from build123d import *

# Parameters (mm, degrees)
F1_DEPTH = 20


with BuildPart() as f1:
    # F0 (on Top) → F1 (new body)
    with BuildSketch(Plane.XY):
        Polygon((1.5, 50), (-1.5, 50), (-1.5, 47), (-1.5, -50), (1.5, -50), (1.5, 27), (51.5, 27), (51.5, 30), (51.5, 50), (48.5, 50), (48.5, 30), (28.5, 30), (28.5, 50), (25.5, 50), (25.5, 30), (1.5, 30), align=None)
    extrude(amount=-F1_DEPTH)

    # F3: sweep along a path in F2
    with BuildLine(Plane(origin=(-1.5, 0, 0), x_dir=(0, -1, 0), z_dir=(-1, 0, 0))) as f3_path:
        Line((-48.5, 0), (-43.5, -20))
    # F0 (on Top) → F3 (sweep)
    with BuildSketch(Plane.XY):
        Polygon((-1.5, 47), (-1.5, 50), (-12, 50), (-12, 47), (-12, 41), (-9, 41), (-5, 41), (-5, 43.5), (-9, 43.5), (-9, 47), align=None)
    sweep(path=f3_path.line)


solid = f1.part
CAD build for the part. Positions are in the model's coordinates, mm. A direction names the side the tool comes from. Round coordinates to 2 decimals unless told otherwise and drop trailing zeros. Write each loop counter-clockwise with the first axis right and the second up, starting at its lowest first coordinate (ties: lowest second). Pieces come first, ordered by that corner, then holes. Notation, with made-up numbers: M 11.25,83.25 L 44.25,83.25 A23 ccw 44.25,92.25 Z; hole C 13.5,-5.75 d4. An arc over 180 degrees is marked long. Use a Markdown table: item, result. Add a question column.
1. Pull direction Z, two halves, no side cores. Call faces 1 (the face through (-7, 41, -10)), 2 (the face through (-6.677, 47.465, -10.14)), 3 (the face through (-1.5, -1, -10)): released by +Z, released by -Z, zero draft, split by the parting line, or undercut.
2. 3-axis set-ups, long thin cutter, end or side, ignore diameter. For faces 4 (the face through (-8.549, 38.465, -10.14)), 5 (the face through (26, 27, -10)), 6 (the face through (39, 30, -10)), 7 (the face through (-5.302, 44.465, -10.14)): which of +Z, -Z, +X, -X, +Y, -Y reach the whole face in a straight line?
3. Slice it at A-A on z = -15. Give the cut face in (x, y), then the cut area to 4 significant figures.
4. Slice it at C-C on y = -19. Give the cut face in (x, z).
5. Flat gauge pins, fed straight in: P1, Ø10, axis at y = -25.5, z = -14, coming from the -X side; P2, Ø2, axis at y = -31.5, z = -12, coming from the +X side; P3, Ø3, axis at x = 7, z = -13.5, coming from the +Y side. Where does each tip first touch, or does it go through?
6. Drill centre lines: probe 1 along X at (y, z) = (37, -11.25); probe 2 along X at (y, z) = (45, -4); probe 3 along X at (y, z) = (23, -10.5). Where is each one in solid material? Low to high.
7. Slice it at B-B on x = 15.5. Give the cut face in (y, z), then the cut area to 3 significant figures.
Reply:
| question | item | result |
|---|---|---|
| 1 | face 1 | undercut |
| 1 | face 2 | released by -Z |
| 1 | face 3 | zero draft |
| 2 | face 4 | +Z, -X, -Y |
| 2 | face 5 | +Z, -Z, +X, -Y |
| 2 | face 6 | +Z, -Z, +Y |
| 2 | face 7 | none |
| 3 | outline | M -12,37.25 L -5,37.25 L -5,39.75 L -9,39.75 L -9,43.25 L -1.5,43.25 L -1.5,-50 L 1.5,-50 L 1.5,27 L 51.5,27 L 51.5,50 L 48.5,50 L 48.5,30 L 28.5,30 L 28.5,50 L 25.5,50 L 25.5,30 L 1.5,30 L 1.5,50 L -1.5,50 L -1.5,46.25 L -12,46.25 Z |
| 3 | area | 629.5 mm^2 |
| 4 | outline | M -1.5,-20 L 1.5,-20 L 1.5,0 L -1.5,0 Z |
| 5 | P1 | stops at x = -1.5 |
| 5 | P2 | stops at x = 1.5 |
| 5 | P3 | stops at y = 30 |
| 6 | probe 1 | x = -1.5 to 1.5, 25.5 to 28.5, 48.5 to 51.5 |
| 6 | probe 2 | x = -12 to -9, -1.5 to 1.5, 25.5 to 28.5, 48.5 to 51.5 |
| 6 | probe 3 | x = -1.5 to 1.5 |
| 7 | outline | M 27,-20 L 30,-20 L 30,0 L 27,0 Z |
| 7 | area | 60.0 mm^2 |
